```python
from build123d import *

# Parameters (mm, degrees)
SKETCH1_W            = 60
SKETCH1_H            = 60
BOSS_EXTRUDE1_DEPTH  = 2
SKETCH2_R            = 1.65
CUT_EXTRUDE1_DEPTH   = 3
LPATTERN1_COUNT      = 6
LPATTERN1_PITCH      = 10
LPATTERN1_COUNT_DIR2 = 6
LPATTERN1_PITCH_DIR2 = 10


with BuildPart() as part:
    # Sketch1 → Boss-Extrude1 (new body)
    with BuildSketch(Plane.XY):
        Rectangle(SKETCH1_W, SKETCH1_H)
    extrude(amount=BOSS_EXTRUDE1_DEPTH)

    # Sketch2 → Cut-Extrude1 (cut, through all)
    with BuildSketch(Plane.XY.offset(2)):
        with Locations((-25, 25)):
            Circle(SKETCH2_R)
    cut_extrude1 = extrude(amount=-CUT_EXTRUDE1_DEPTH, mode=Mode.SUBTRACT)

    # LPattern1: Cut-Extrude1 6 × 6
    with Locations(*[(j * LPATTERN1_PITCH_DIR2, -i * LPATTERN1_PITCH, 0) for i in range(LPATTERN1_COUNT) for j in range(LPATTERN1_COUNT_DIR2) if (i, j) != (0, 0)]):
        add(cut_extrude1, mode=Mode.SUBTRACT)


solid = part.part
```
Verification items for the finished model (mm, model axes). Coordinates: 2 decimals unless noted, no trailing zeros. Loops run counter-clockwise (first coordinate to the right, second up) from the corner with the lowest first, then second, coordinate; pieces in that order, holes last. Notation, with made-up numbers: (-9, 47.5) - (22, 47.5) arc R25 ccw to (22, 65.5) - close; hole circle Ø7 at (-32.75, 8.25). An arc over 180 degrees is marked (long way). Answer as a JSON object with one key per item and string values.
(1) Cross-section at C-C, the plane z = 1.05. Count the separate pieces of the cut face and the enclosed holes in it, then the cut area to 3 significant figures.
Response:
{"separate pieces": "1", "enclosed holes": "36", "area": "3,290 mm²"}
(2) Cross-section at A-A, the plane x = 5. Record the boundary of the cut face in (y, z), then the cut area to 3 significant figures.
Response:
{"outline": "(-30, 0) - (-26.65, 0) - (-26.65, 2) - (-30, 2) - close; (-23.35, 0) - (-16.65, 0) - (-16.65, 2) - (-23.35, 2) - close; (-13.35, 0) - (-6.65, 0) - (-6.65, 2) - (-13.35, 2) - close; (-3.35, 0) - (3.35, 0) - (3.35, 2) - (-3.35, 2) - close; (6.65, 0) - (13.35, 0) - (13.35, 2) - (6.65, 2) - close; (16.65, 0) - (23.35, 0) - (23.35, 2) - (16.65, 2) - close; (26.65, 0) - (30, 0) - (30, 2) - (26.65, 2) - close", "area": "80.4 mm²"}
(3) Go/stop test with a flat-tipped pin: pin 1 Ø2.5 at (x, y) = (-15, -25) entering from +Z. Record where the tip stops, or that it passes through.
Response:
{"pin 1": "passes through"}
(4) Mould release check, pull along Y, two halves, no side actions. Record for faces 1 (the cylindrical face through (-5.215, -23.364, 1.014)), 2 (the flat face through (0, 30, 1)), 3 (the flat face through (-30, 0, 1)): pulls with the +Y half, pulls with the -Y half, needs draft (parallel to the pull), parting line crosses it, or undercut.
Response:
{"face 1": "undercut", "face 2": "pulls with the +Y half", "face 3": "needs draft"}
